Study the drawing (mm; zero at the part's minimum x, y, z) and answer. Coordinates: 2 decimals unless noted, no trailing zeros. Order: outer loops, then holes, each group sorted by start corner. A loop starts at its lowest first (then second) coordinate and runs counter-clockwise, first axis right, second up. Notation, with made-up numbers: (87, 11) -> (95, 11) arc R30 ccw to (95, 49) -> close; hole circle Ø8 at (68.5, 5.25). An arc over 180 degrees is marked (long way). One line per question, with ' | ' between items.
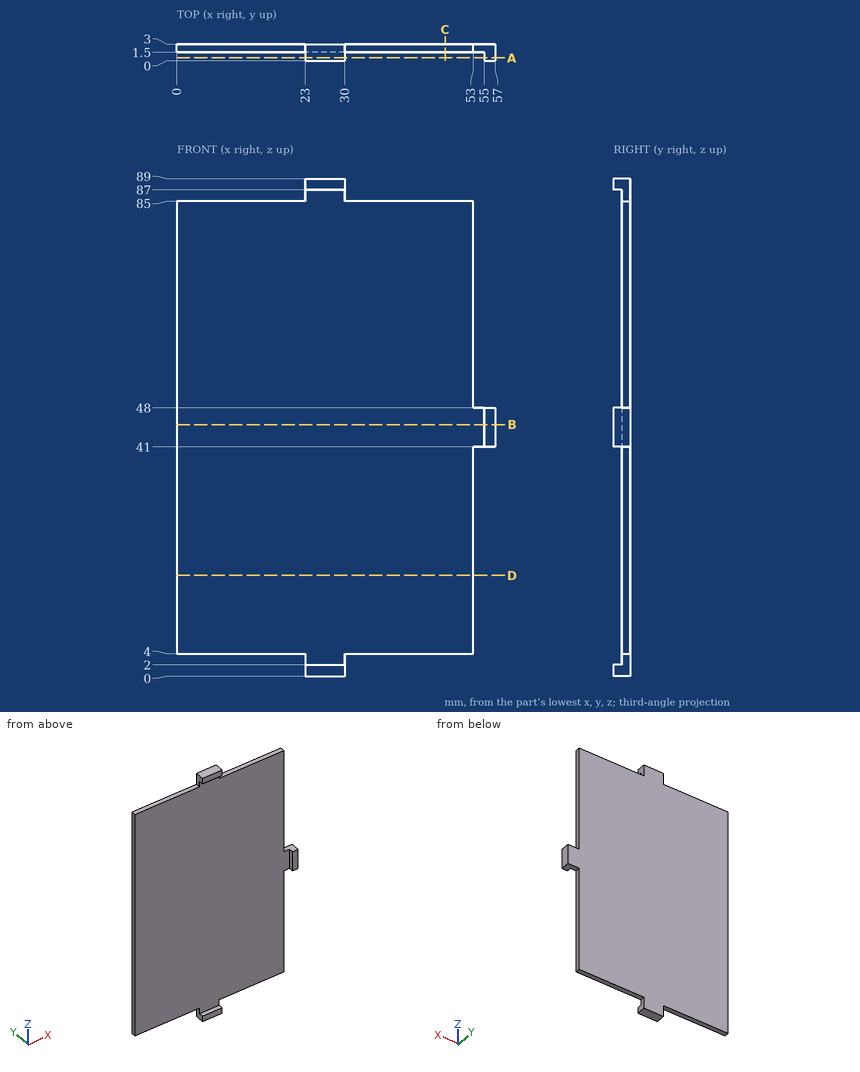
Item 1: Section A-A, the plane y = 0.5 is taken. Give the vertices of the cut face in (x, z).
Computed values:
outline: (23, 0) -> (30, 0) -> (30, 2) -> (23, 2) -> close; (23, 87) -> (30, 87) -> (30, 89) -> (23, 89) -> close; (55, 41) -> (57, 41) -> (57, 48) -> (55, 48) -> close
Item 2: Each of these flat-tipped pins is pushed along its axis until it touches: pin 1 Ø0.8 at (x, y) = (15.5, 2) entering from +Z; pin 2 Ø1.2 at (y, z) = (2.5, 62.5) entering from +X; pin 3 Ø8 at (x, z) = (39, 43.5) entering from -Y. Where does it stop, or does it pass through?
Computed values:
pin 1: stops at z = 85 | pin 2: stops at x = 53 | pin 3: stops at y = 1.5
Item 3: Section D-D, the plane z = 18 is taken. Give the vertices of the cut face in (x, y), plus the area to 3 significant figures.
Computed values:
outline: (0, 1.5) -> (53, 1.5) -> (53, 3) -> (0, 3) -> close | area: 79.5 mm^2
Item 4: Find the intervals of material crossed by L1, parallel to Z at x = 24.5, y = 1.35; L2, parallel to Z at x = 43, y = 2.4; L3, parallel to Y at x = 5.5, z = 52.5, in increasing order.
Computed values:
L1: z = 0 to 2, 87 to 89 | L2: z = 4 to 85 | L3: y = 1.5 to 3
Item 5: Section C-C, the plane x = 48 is taken. Give the vertices of the cut face in (y, z), plus the area to 4 significant figures.
Computed values:
outline: (1.5, 4) -> (3, 4) -> (3, 85) -> (1.5, 85) -> close | area: 121.5 mm^2
Item 6: Section B-B, the plane z = 45 is taken. Give the vertices of the cut face in (x, y).
Computed values:
outline: (0, 1.5) -> (55, 1.5) -> (55, 0) -> (57, 0) -> (57, 3) -> (0, 3) -> close
